Design review of the part shown in the three views and the two pictorial views. Dimensions are in mm from the part's minimum x, y and z. Coordinates: 2 decimals unless noted, no trailing zeros. Loops run counter-clockwise (first coordinate to the right, second up) from the corner with the lowest first, then second, coordinate; pieces in that order, holes last. Notation, with made-up numbers: (2, -25) -> (31, -25) arc R15 ccw to (31, -10) -> close; hole circle Ø10 at (71.5, 43). An arc over 180 degrees is marked (long way). One line per item, written item: value.
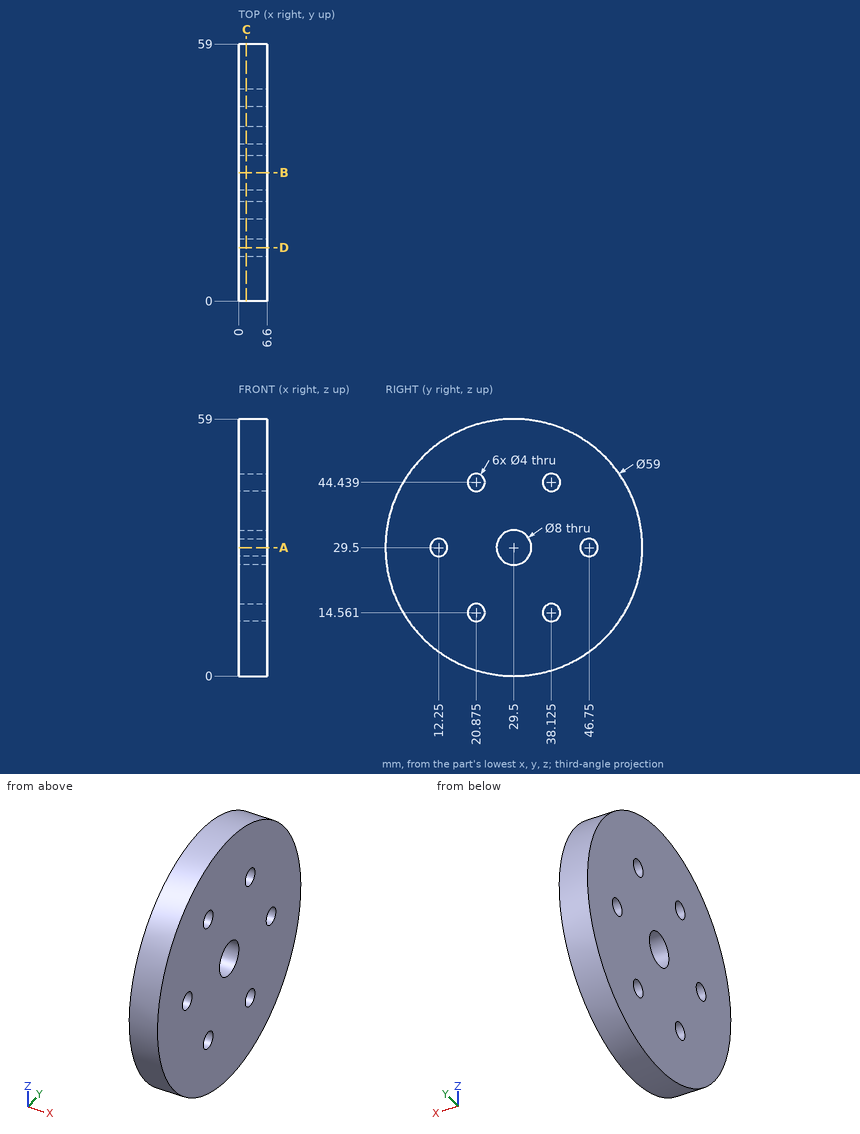
1. Take a section at C-C, the plane x = 1.75. Give the boundary of the cut face in (y, z) (3 decimals).
Return value:
outline: circle Ø59 at (29.5, 29.5); hole circle Ø4 at (12.25, 29.5); hole circle Ø4 at (20.875, 14.561); hole circle Ø4 at (20.875, 44.439); hole circle Ø8 at (29.5, 29.5); hole circle Ø4 at (38.125, 14.561); hole circle Ø4 at (38.125, 44.439); hole circle Ø4 at (46.75, 29.5)
2. Take a section at A-A, the plane z = 29.5. Give the boundary of the cut face in (x, y), and give its area (3 significant figures).
Return value:
outline: (0, 0) -> (6.6, 0) -> (6.6, 10.25) -> (0, 10.25) -> close; (0, 14.25) -> (6.6, 14.25) -> (6.6, 25.5) -> (0, 25.5) -> close; (0, 33.5) -> (6.6, 33.5) -> (6.6, 44.75) -> (0, 44.75) -> close; (0, 48.75) -> (6.6, 48.75) -> (6.6, 59) -> (0, 59) -> close
area: 284 mm2
3. To check wall thickness, follow probe 1 along Y at (x, z) = (2, 29.5); probe 2 along Y at (x, z) = (6.25, 46) (1 decimal); probe 3 along Y at (x, z) = (3.25, 45). State the ranges of each line that lie inside material, in increasing order. Write a range as from..to.
Return value:
probe 1: y = 0..10.25, 14.25..25.5, 33.5..44.75, 48.75..59
probe 2: y = 5..19.6, 22.1..36.9, 39.4..54
probe 3: y = 4.4..18.96, 22.79..36.21, 40.04..54.6
4. Take a section at D-D, the plane y = 12.25. Give the boundary of the cut face in (x, z), and give its area (4 significant figures).
Return value:
outline: (0, 5.57) -> (6.6, 5.57) -> (6.6, 27.5) -> (0, 27.5) -> close; (0, 31.5) -> (6.6, 31.5) -> (6.6, 53.43) -> (0, 53.43) -> close
area: 289.5 mm2
5. Insertion check: pin 1 Ø3 at (x, z) = (3, 25) entering from +Y; pin 2 Ø5 at (y, z) = (29.5, 29.5) entering from -X; pin 3 Ø1 at (x, y) = (2.5, 36) entering from +Z. Each pin has a flat end and moves straight along its axis. Give the tip position at first contact, or say it passes through.
Return value:
pin 1: stops at y = 58.85
pin 2: passes through
pin 3: stops at z = 58.38
6. Take a section at B-B, the plane y = 29.5. Give the boundary of the cut face in (x, z).
Return value:
outline: (0, 0) -> (6.6, 0) -> (6.6, 25.5) -> (0, 25.5) -> close; (0, 33.5) -> (6.6, 33.5) -> (6.6, 59) -> (0, 59) -> close
